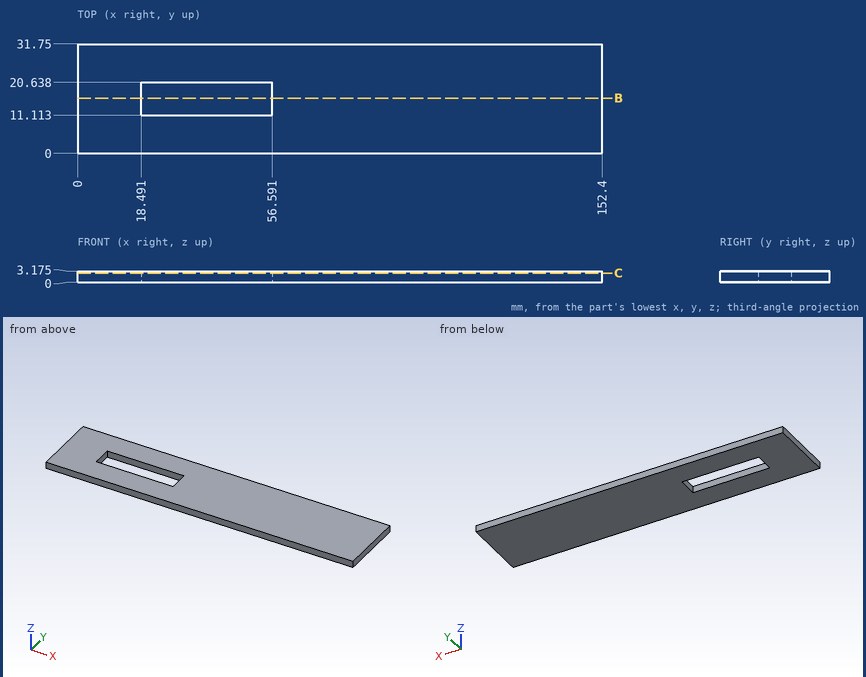
Job drawing, mm, ordinate dimensions from the low corner. One solid piece. Round coordinates to 2 decimals unless told otherwise and drop trailing zeros. Write each loop counter-clockwise with the first axis right and the second up, starting at its lowest first coordinate (ties: lowest second). Pieces come first, ordered by that corner, then holes. Notation, with made-up numbers: M 53.25,-27 L 63.25,-27 A12 ccw 63.25,-8 Z; hole C -33.75,85.5 d9. An arc over 180 degrees is marked long. Return JSON: item names as keys, results as strings. Group by question number.
(1) Saw through at B-B on y = 16. Write the cut outline in (x, z) (1 decimal), then the cut area to 3 significant figures.
(2) Saw through at C-C on z = 2.65. Write the cut outline in (x, y).
(3) Drill centre lines: probe 1 along X at (y, z) = (12.5, 2.85); probe 2 along Y at (x, z) = (26.5, 0.2). Where is each one in solid material? Low to high.
Returned:
{
 "1": {"outline": "M 0,0 L 18.5,0 L 18.5,3.2 L 0,3.2 Z; M 56.6,0 L 152.4,0 L 152.4,3.2 L 56.6,3.2 Z", "area": "363 mm²"},
 "2": {"outline": "M 0,0 L 152.4,0 L 152.4,31.75 L 0,31.75 Z; hole M 18.49,11.11 L 56.59,11.11 L 56.59,20.64 L 18.49,20.64 Z"},
 "3": {"probe 1": "0 to 18.49, 56.59 to 152.4", "probe 2": "0 to 11.11, 20.64 to 31.75"}
}
